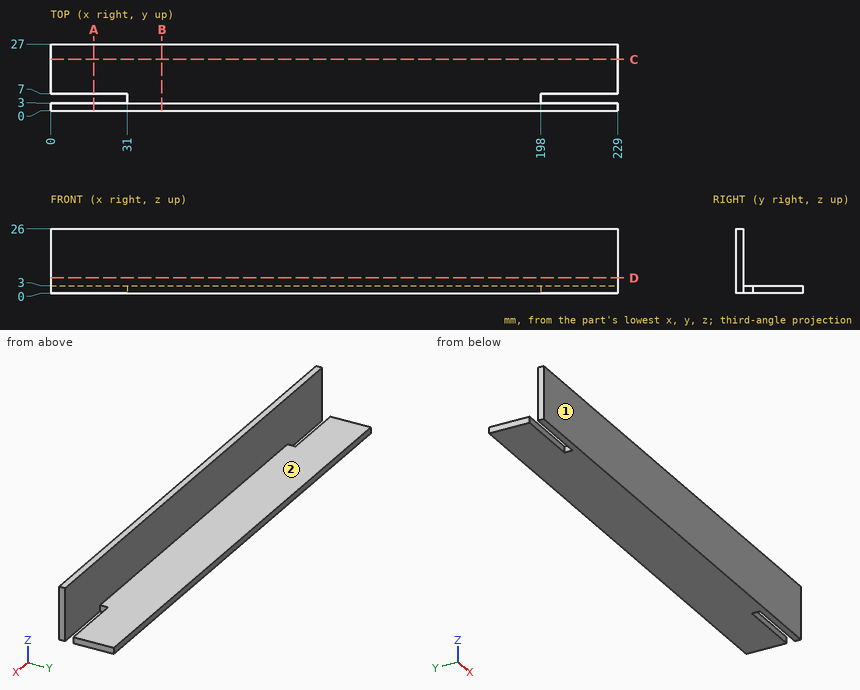
The figure shows three views and two pictorial views of one solid part (mm, origin at its lowest corner). Answer the questions. A direction names the side the tool comes from. Coordinates: 2 decimals unless noted, no trailing zeros. Loops run counter-clockwise (first coordinate to the right, second up) from the corner with the lowest first, then second, coordinate; pieces in that order, holes last.
1) A tool of negligible diameter and unlimited length cuts with its end or side. For the marked faces 1 and 2, from which of +Z, -Z, +X, -X, +Y, -Y can it reach the whole face along a straight path? Write none if from no direction.
2) Flat-ended cylindrical pins translate along their axes: pin 1 Ø1.5 at (y, z) = (4, 1) entering from -X; pin 2 Ø3 at (x, z) = (158, 5.5) entering from +Y; pin 3 Ø1.5 at (x, z) = (8, 2) entering from -Y; pin 4 Ø2.5 at (y, z) = (5.5, 2) entering from +X. Find the tip coordinate at first contact, or state that the pin passes through.
3) Find section A-A on x = 17.5. Write down the section's boundary in (y, z).
4) Find section B-B on x = 45. Write down the section's boundary in (y, z), then the cut area to 3 significant figures.
5) Find section C-C on y = 20.75. Write down the section's boundary in (x, z).
6) Find the intervals of material crossed by L1, parallel to Y at x = 29.5, z = 1.5; L2, parallel to Y at x = 137, z = 12.5, in increasing order.
Values:
1. face 1: +Z, -Z, +X, -X, -Y
1. face 2: +Z, +X, -X, +Y
2. pin 1: stops at x = 31
2. pin 2: stops at y = 3
2. pin 3: stops at y = 0
2. pin 4: stops at x = 198
3. outline: (0, 0) - (3, 0) - (3, 26) - (0, 26) - close; (7, 0) - (27, 0) - (27, 3) - (7, 3) - close
4. outline: (0, 0) - (27, 0) - (27, 3) - (3, 3) - (3, 26) - (0, 26) - close
4. area: 150 mm2
5. outline: (0, 0) - (229, 0) - (229, 3) - (0, 3) - close
6. L1: y = 0 to 3, 7 to 27
6. L2: y = 0 to 3
